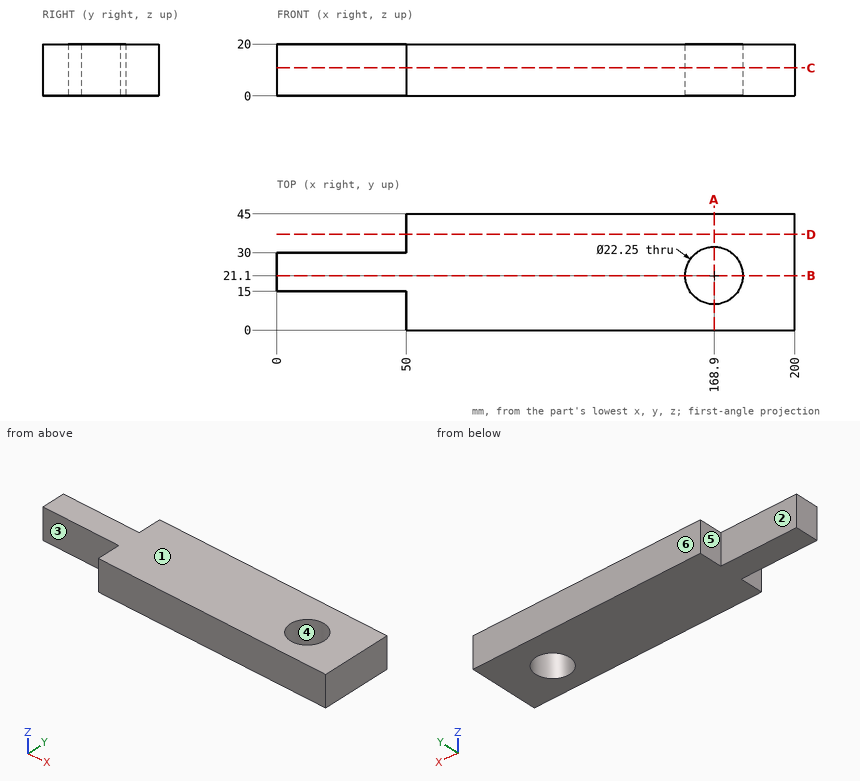
For this review, use the dimensioned drawing (mm, ordinates from the lowest corner) and the shaded views. A direction names the side the tool comes from. Give positions to 0.01 mm unless a question says otherwise; leave off trailing zeros. Write each loop counter-clockwise with the first axis right and the second up, starting at its lowest first coordinate (ties: lowest second). Pieces come first, ordered by that corner, then holes. Notation, with made-up numbers: M 8,58 L 33,58 A19 cw 33,76 Z; hole C 2.5,85 d5. An arc over 180 degrees is marked long. Answer as a JSON object with one key per item and string values. Group by question number.
1) We need section B-B (y = 21.1). Give the boundary of the cut face in (x, z) (3 decimals), and give its area (4 significant figures).
2) We need section C-C (z = 10.75). Give the boundary of the cut face in (x, y) (3 decimals), and give its area (3 significant figures).
3) Clearance check with flat-ended pins moving along their axes: pin 1 Ø10 at (x, z) = (35.5, 6.5) entering from -Y; pin 2 Ø3 at (x, z) = (34.5, 17) entering from +Y; pin 3 Ø2 at (y, z) = (10.5, 17.5) entering from -X. State where each tip first meets the part, or that it passes through.
4) For line 1 along Y through (x, z) = (168.9, 5.25) (3 decimals); line 2 along X through (y, z) = (21, 16.75); line 3 along X through (y, z) = (2.5, 12.5), list the stretches that pass through material, from the lowest coordinate up.
5) Tool access review of the marked faces 1, 2 and 3: name each direction out of +Z, -Z, +X, -X, +Y, -Y from which nothing blocks a thin tool from reaching the whole face with its end or side.
6) Mouldability with a two-part tool opening along Y and no side actions: class the marked faces 4, 5 and 6 as released by +Y, released by -Y, zero draft, split by the parting line, or undercut.
7) We need section A-A (x = 168.9). Give the boundary of the cut face in (y, z) (3 decimals), and give its area (3 significant figures).
8) We need section D-D (y = 37). Give the boundary of the cut face in (x, z), and give its area (3 significant figures).
Answer key:
{
 "1": {"outline": "M 0,0 L 157.775,0 L 157.775,20 L 0,20 Z; M 180.025,0 L 200,0 L 200,20 L 180.025,20 Z", "area": "3,555 mm²"},
 "2": {"outline": "M 0,15 L 50,15 L 50,0 L 200,0 L 200,45 L 50,45 L 50,30 L 0,30 Z; hole C 168.9,21.1 d22.25", "area": "7,110 mm²"},
 "3": {"pin 1": "stops at y = 15", "pin 2": "stops at y = 30", "pin 3": "stops at x = 50"},
 "4": {"line 1": "y = 0 to 9.975, 32.225 to 45", "line 2": "x = 0 to 157.78, 180.02 to 200", "line 3": "x = 50 to 200"},
 "5": {"face 1": "+Z, +X, -X, +Y, -Y", "face 2": "+Z, -Z, -X, +Y", "face 3": "+Z, -Z, -X, -Y"},
 "6": {"face 4": "undercut", "face 5": "zero draft", "face 6": "released by +Y"},
 "7": {"outline": "M 0,0 L 9.975,0 L 9.975,20 L 0,20 Z; M 32.225,0 L 45,0 L 45,20 L 32.225,20 Z", "area": "455 mm²"},
 "8": {"outline": "M 50,0 L 200,0 L 200,20 L 50,20 Z", "area": "3,000 mm²"}
}
